The model under review builds one solid part; all positions refer to its coordinate system, in mm. A direction names the side the tool comes from. Give positions to 0.01 mm unless a question says otherwise; leave off trailing zeros. Write each loop counter-clockwise with the first axis right and the second up, starting at its lowest first coordinate (ties: lowest second). Pieces come first, ordered by that corner, then holes. Notation, with made-up numbers: (-28.5, -18.75) - (23.5, -18.75) arc R26 ccw to (23.5, 0.25) - close; hole circle Ø4 at (30.5, 7). An arc over 180 degrees is marked (long way). Write item = value, one per line.
```python
from build123d import *

# Parameters (mm, degrees)
SALIENTE_EXTRUIR1_DEPTH = 80
CROQUIS2_R              = 2.5
CORTAR_EXTRUIR1_DEPTH   = 99.111161445
CROQUIS3_R              = 2.5
CORTAR_EXTRUIR2_DEPTH   = 99.111161445
CROQUIS4_W              = 30
CROQUIS4_H              = 10
CORTAR_EXTRUIR3_DEPTH   = 99.111161445


with BuildPart() as part:
    # Croquis1 → Saliente-Extruir1 (new body)
    with BuildSketch(Plane(origin=(0, 0, 0), x_dir=(1, 0, 0), z_dir=(0, 1, 0))):
        Polygon((25.4, 0), (0, 0), (0, 50.8), (3.175, 50.8), (3.175, 3.175), (25.4, 3.175), align=None)
    extrude(amount=SALIENTE_EXTRUIR1_DEPTH)

    # Croquis2 → Cortar-Extruir1 (cut, through all)
    with BuildSketch(Plane.ZY):
        with Locations((-41.3, 67.5)):
            Circle(CROQUIS2_R)
        with Locations((-20.3, 67.5)):
            Circle(CROQUIS2_R)
        with Locations((-20.3, 12.5)):
            Circle(CROQUIS2_R)
        with Locations((-41.3, 12.5)):
            Circle(CROQUIS2_R)
    extrude(amount=-CORTAR_EXTRUIR1_DEPTH, mode=Mode.SUBTRACT)

    # Croquis3 → Cortar-Extruir2 (cut, through all)
    with BuildSketch(Plane.XY):
        with Locations((12.7, 70)):
            Circle(CROQUIS3_R)
        with Locations((12.7, 10)):
            Circle(CROQUIS3_R)
    extrude(amount=-CORTAR_EXTRUIR2_DEPTH, mode=Mode.SUBTRACT)

    # Croquis4 → Cortar-Extruir3 (cut, through all)
    with BuildSketch(Plane.XY):
        with Locations((12.7, 0)):
            Rectangle(CROQUIS4_W, CROQUIS4_H)
    extrude(amount=-CORTAR_EXTRUIR3_DEPTH, mode=Mode.SUBTRACT)


solid = part.part
```
1. Take a section at D-D on y = 34.5. Give the boundary of the cut face in (x, z) (3 decimals), and give its area (3 significant figures).
Findings below:
outline = (0, -50.8) - (3.175, -50.8) - (3.175, -3.175) - (25.4, -3.175) - (25.4, 0) - (0, 0) - close
area = 232 mm²
2. Take a section at A-A on x = 12.7. Give the boundary of the cut face in (y, z) (3 decimals), and give its area (3 significant figures).
Findings below:
outline = (5, -3.175) - (7.5, -3.175) - (7.5, 0) - (5, 0) - close; (12.5, -3.175) - (67.5, -3.175) - (67.5, 0) - (12.5, 0) - close; (72.5, -3.175) - (80, -3.175) - (80, 0) - (72.5, 0) - close
area = 206 mm²
3. Take a section at C-C on z = -41.3. Give the boundary of the cut face in (x, y) (3 decimals).
Findings below:
outline = (0, 5) - (3.175, 5) - (3.175, 10) - (0, 10) - close; (0, 15) - (3.175, 15) - (3.175, 65) - (0, 65) - close; (0, 70) - (3.175, 70) - (3.175, 80) - (0, 80) - close
4. Insertion check: P1, Ø4, axis at x = 12.7, y = 70, coming from the +Z side; P2, Ø3, axis at x = 13, y = 42.5, coming from the +Z side; P3, Ø6.5, axis at x = 19, y = 30.5, coming from the -Z side (3 decimals); P4, Ø2, axis at y = 27.5, z = -18, coming from the +X side (3 decimals). Each pin has a flat end and moves straight along its axis. Give the tip position at first contact, or say it passes through.
Findings below:
P1 = through
P2 = 0
P3 = -3.175
P4 = 3.175
5. For line 1 (Y direction, x = 12.7, z = -2); line 2 (Y direction, x = 1.7, z = -20.3); line 3 (X direction, y = 72.5, z = -15) (3 decimals), list the stretches that pass through material, from the lowest coordinate up. Write a range as from..to.
Findings below:
line_1 = 5..7.5, 12.5..67.5, 72.5..80
line_2 = 5..10, 15..65, 70..80
line_3 = 0..3.175
6. Take a section at B-B on y = 14. Give the boundary of the cut face in (x, z) (3 decimals).
Findings below:
outline = (0, -50.8) - (3.175, -50.8) - (3.175, -43.3) - (0, -43.3) - close; (0, -39.3) - (3.175, -39.3) - (3.175, -22.3) - (0, -22.3) - close; (0, -18.3) - (3.175, -18.3) - (3.175, -3.175) - (25.4, -3.175) - (25.4, 0) - (0, 0) - close
7. Machinability: for faces 4 (the flat face through (3.175, 42, -27)), 5 (the cylindrical face through (1.6, 12.6, -43.8)), which of the approach directions +Z, -Z, +X, -X, +Y, -Y give a long, thin tool a straight path to every point of the face, cutting with its end or side? Answer none if there is none.
Findings below:
face_4 = -Z, +X, +Y, -Y
face_5 = +X, -X
8. Draft analysis for pull direction Z (two halves, no side actions). For faces 1 (the flat face through (2, 80, -16)), 2 (the flat face through (2, 42, -50.8)), 3 (the cylindrical face through (1.57, 10.06, -20.84)), state which applies: +Z half, -Z half, draft (parallel to the pull), parting line (faces both ways), or undercut.
Findings below:
face_1 = draft
face_2 = -Z half
face_3 = undercut
